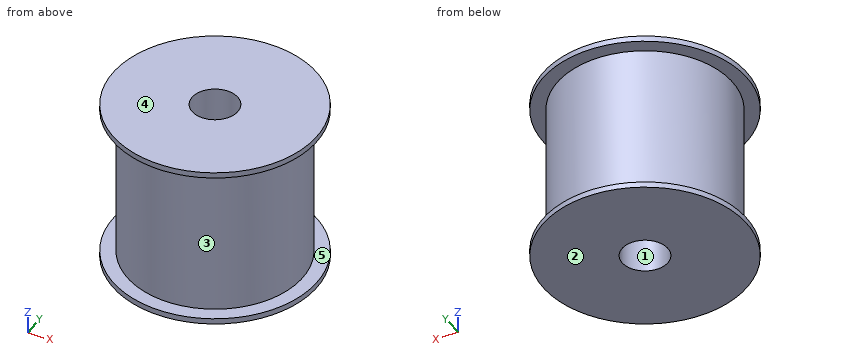
```python
from build123d import *

# Parameters (mm, degrees)
SKETCH1_R           = 15.3
BOSS_EXTRUDE1_DEPTH = 27
SKETCH2_R           = 17.8
BOSS_EXTRUDE2_DEPTH = 1
BOSS_EXTRUDE4_START = 1
SKETCH6_R           = 17.8
BOSS_EXTRUDE4_DEPTH = 1
SKETCH7_R           = 4
CUT_EXTRUDE1_DEPTH  = 39.401562468


with BuildPart() as part:
    # Sketch1 → Boss-Extrude1 (new body)
    with BuildSketch(Plane.XY):
        Circle(SKETCH1_R)
    extrude(amount=BOSS_EXTRUDE1_DEPTH)

    # Sketch2 → Boss-Extrude2 (add)
    with BuildSketch(Plane.XY.offset(27)):
        Circle(SKETCH2_R)
    extrude(amount=BOSS_EXTRUDE2_DEPTH)

    # Sketch6 → Boss-Extrude4 (add)
    with BuildSketch(Plane(origin=(0, 0, 0), x_dir=(-1, 0, 0), z_dir=(0, 0, -1)).offset(BOSS_EXTRUDE4_START)):
        with Locations(Location((0, 0, 0), (0, 0, 180))):
            Circle(SKETCH6_R)
    extrude(amount=-BOSS_EXTRUDE4_DEPTH)

    # Sketch7 → Cut-Extrude1 (cut, through all)
    with BuildSketch(Plane(origin=(0, 0, -1), x_dir=(-1, 0, 0), z_dir=(0, 0, -1))):
        Circle(SKETCH7_R)
    extrude(amount=-CUT_EXTRUDE1_DEPTH, mode=Mode.SUBTRACT)


solid = part.part
```
Can you work these out from the model? Positions are in its coordinate system, mm. Face numbers are marked on the shaded views. A direction names the side the tool comes from. Give positions to 0.01 mm unless a question says otherwise; leave off trailing zeros. Loops run counter-clockwise (first coordinate to the right, second up) from the corner with the lowest first, then second, coordinate; pieces in that order, holes last. Notation, with made-up numbers: M 18,-4 L 41,-4 A28 cw 41,32 Z; hole C -24,-19.5 d5. An arc over 180 degrees is marked long. One line per question, with ' | ' between items. Start each with the question number.
Q1. If we section it at D-D (x = -8): Please give me the cut outline in (y, z), plus the area to 3 significant figures.
Q2. If we section it at C-C (z = 13.75): Please give me the cut outline in (x, y), plus the area to 3 significant figures.
Q3. If I drill on line 1 (Y direction, x = 0, z = 6.25); line 2 (Z direction, x = -11, y = -11); line 3 (Y direction, x = -1, z = 3), over which ranges is the centre line in solid material (lowest first)? Write a range as from..to.
Q4. If we section it at A-A (y = 0): Please give me the cut outline in (x, z).
Q5. For the marked faces 4 and 5, which set-ups out of +Z, -Z, +X, -X, +Y, -Y let a thin tool reach every point of the face, with its end or its side?
Q6. If we mould it in two halves opening along Z, with no side actions, what happens to the marked faces 1, 2 and 3? For each: +Z half, -Z half, draft (parallel to the pull), parting line (faces both ways), or undercut.
Q7. For pin 1 Ø12 at (x, z) = (-3.5, 8.5) entering from +Y; pin 2 Ø8 at (x, z) = (-3, 4.5) entering from -Y; pin 3 Ø5 at (x, y) = (0, 0) entering from +Z; pin 4 Ø3 at (y, z) = (-5, 7.5) entering from +X, each with a flat end and sliding along its axis, tell me the tip position at first contact or that it passes through.
Computed:
1) outline: M -15.9,-1 L 15.9,-1 L 15.9,0 L 13.04,0 L 13.04,27 L 15.9,27 L 15.9,28 L -15.9,28 L -15.9,27 L -13.04,27 L -13.04,0 L -15.9,0 Z | area: 768 mm²
2) outline: C 0,0 d30.6; hole C 0,0 d8 | area: 685 mm²
3) line 1: y = -15.3..-4, 4..15.3 | line 2: z = -1..0, 27..28 | line 3: y = -15.27..-3.87, 3.87..15.27
4) outline: M -17.8,-1 L -4,-1 L -4,28 L -17.8,28 L -17.8,27 L -15.3,27 L -15.3,0 L -17.8,0 Z; M 4,-1 L 17.8,-1 L 17.8,0 L 15.3,0 L 15.3,27 L 17.8,27 L 17.8,28 L 4,28 Z
5) face 4: +Z, +X, -X, +Y, -Y | face 5: none
6) face 1: draft | face 2: -Z half | face 3: undercut
7) pin 1: stops at y = 15.3 | pin 2: stops at y = -15.3 | pin 3: passes through | pin 4: stops at x = 14.89
